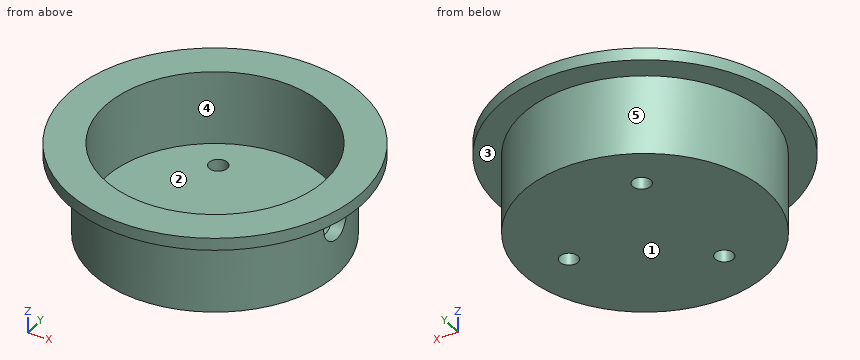
from build123d import *

# Parameters (mm, degrees)
SKETCH_3_R          = 3
CUT_EXTRUDE_1_DEPTH = 75.215901261
SKETCH_4_R          = 6
CUT_EXTRUDE_2_DEPTH = 6


with BuildPart() as part:
    # 草图2 → 旋转2 (revolve)
    with BuildSketch(Plane(origin=(0, 0, 0), x_dir=(1, 0, 0), z_dir=(0, 1, 0)), mode=Mode.PRIVATE) as revolve_2_sk:
        Polygon((0, 0), (40, 0), (40, -26), (48, -26), (48, -30), (36, -30), (36, -6), (0, -6), align=None)
    revolve(revolve_2_sk.sketch.rotate(Axis((0, 0, 0), (0, 0, 1)), 180), axis=Axis((0, 0, 0), (0, 0, 1)))

    # 草图3 → 切除-拉伸1 (cut, through all)
    with BuildSketch(Plane.XY):
        with Locations(Location((25, 0, 0), (0, 0, 180))):
            Circle(SKETCH_3_R)
        with Locations(Location((-12.5, 21.650635, 0), (0, 0, 180))):
            Circle(SKETCH_3_R)
        with Locations(Location((-12.5, -21.650635, 0), (0, 0, 180))):
            Circle(SKETCH_3_R)
    extrude(amount=CUT_EXTRUDE_1_DEPTH, mode=Mode.SUBTRACT)

    # 草图4 → 切除-拉伸2 (cut)
    with BuildSketch(Plane(origin=(40, 0, 0), x_dir=(0, 0, -1), z_dir=(1, 0, 0))):
        with Locations((-18, 0)):
            Circle(SKETCH_4_R)
    extrude(amount=-CUT_EXTRUDE_2_DEPTH, mode=Mode.SUBTRACT)


solid = part.part
Read the model definition and answer for the solid it produces. Units are mm, in the model's axes. Face numbers are marked on the shaded views. A direction names the side the tool comes from. Give positions to 0.01 mm unless a question says otherwise; leave off trailing zeros. Write each loop counter-clockwise with the first axis right and the second up, starting at its lowest first coordinate (ties: lowest second). Pieces come first, ordered by that corner, then holes. Notation, with made-up numbers: M 24,69 L 55,69 A16 ccw 55,90 Z; hole C 54.5,82.5 d8. An arc over 180 degrees is marked long. One line per item, written item: value. Start each with the question number.
(1) Find section D-D (x = -12.5). Determine the outline of the cut face in (y, z).
(2) Find the intervals of material crossed by line 1 (Y direction, x = 0, z = 18.5); line 2 (Z direction, x = -21, y = -40.5); line 3 (Y direction, x = -12, z = 2), in increasing order.
(3) A tool of negligible diameter and unlimited length cuts with its end or side. For the marked faces 1 and 2, from which of +Z, -Z, +X, -X, +Y, -Y can it reach the whole face along a straight path? Write none if from no direction.
(4) Flat-ended cylindrical pins translate along their axes: pin 1 Ø1 at (y, z) = (-36.5, 24) entering from -X; pin 2 Ø8 at (y, z) = (29.5, 12) entering from +X; pin 3 Ø3 at (y, z) = (15, 21.5) entering from -X; pin 4 Ø5.5 at (x, y) = (25, 0) entering from -Z. Find the tip coordinate at first contact, or state that the pin passes through.
(5) Find section C-C (y = 20). Determine the outline of the cut face in (x, z).
(6) Find section B-B (x = 25). Determine the outline of the cut face in (y, z), plus the area to 3 significant figures.
(7) Determine the mould class of the marked faces 3, 4 and 5 for opening direction X: pulls with the +X half, pulls with the -X half, needs draft (parallel to the pull), parting line crosses it, or undercut.
(8) Find section A-A (y = 0). Determine the outline of the cut face in (x, z).
Results below:
1. outline: M -46.34,26 L -38,26 L -38,0 L -24.65,0 L -24.65,6 L -33.76,6 L -33.76,30 L -46.34,30 Z; M -18.65,0 L 18.65,0 L 18.65,6 L -18.65,6 Z; M 24.65,0 L 38,0 L 38,26 L 46.34,26 L 46.34,30 L 33.76,30 L 33.76,6 L 24.65,6 Z
2. line 1: y = -40 to -36, 36 to 40
2. line 2: z = 26 to 30
2. line 3: y = -38.16 to -24.61, -18.69 to 18.69, 24.61 to 38.16
3. face 1: -Z, +X, -X, +Y, -Y
3. face 2: +Z
4. pin 1: stops at x = -17.44
4. pin 2: stops at x = 30.82
4. pin 3: stops at x = -37.65
4. pin 4: passes through
5. outline: M -43.63,26 L -34.64,26 L -34.64,0 L -15.01,0 L -15.01,6 L -29.93,6 L -29.93,30 L -43.63,30 Z; M -9.99,0 L 34.64,0 L 34.64,26 L 43.63,26 L 43.63,30 L 29.93,30 L 29.93,6 L -9.99,6 Z
6. outline: M -40.98,26 L -31.22,26 L -31.22,0 L -3,0 L -3,6 L -25.9,6 L -25.9,30 L -40.98,30 Z; M 3,0 L 31.22,0 L 31.22,26 L 40.98,26 L 40.98,30 L 25.9,30 L 25.9,6 L 3,6 Z
6. area: 672 mm^2
7. face 3: needs draft
7. face 4: undercut
7. face 5: parting line crosses it
8. outline: M -48,26 L -40,26 L -40,0 L 22,0 L 22,6 L -36,6 L -36,30 L -48,30 Z; M 28,0 L 40,0 L 40,12 L 36,12 L 36,6 L 28,6 Z; M 36,24 L 40,24 L 40,26 L 48,26 L 48,30 L 36,30 Z
